Input: dimensioned drawing with shaded views. Units: mm. Origin: part minimum x, y, z. Round coordinates to 2 decimals unless told otherwise and drop trailing zeros. Loops run counter-clockwise (first coordinate to the right, second up) from the corner with the lowest first, then second, coordinate; pieces in that order, holes last. Notation, with made-up numbers: M 23,14 L 69,14 A15 cw 69,24 Z; hole C 62,-22 d4. An arc over 180 degrees is marked long. Use one line per item in the form item = value. Start each with the question number.
Q1. Section query A-A, the plane z = 16.51. Output: boundary loops of the cut face in (x, y), and give its area (3 significant figures).
Q2. Section query B-B, the plane x = 35.56. Output: boundary loops of the cut face in (y, z), and give its area (3 significant figures).
Q3. Ray query, line 1 along X through (y, z) = (0.95, 16.51); line 2 along Z through (x, y) = (22, 1.8); line 3 along X through (y, z) = (0.55, 18.5). Return the intervals inside material, ascending.
Q4. Section query C-C, the plane y = 0.5. Output: boundary loops of the cut face in (x, z).
Q5. First-contact query: P1, Ø24.5, axis at x = 35.56, z = 16.51, coming from the +Y side. Flat tip, straight axial feed; report the tip coordinate or a pass-through.
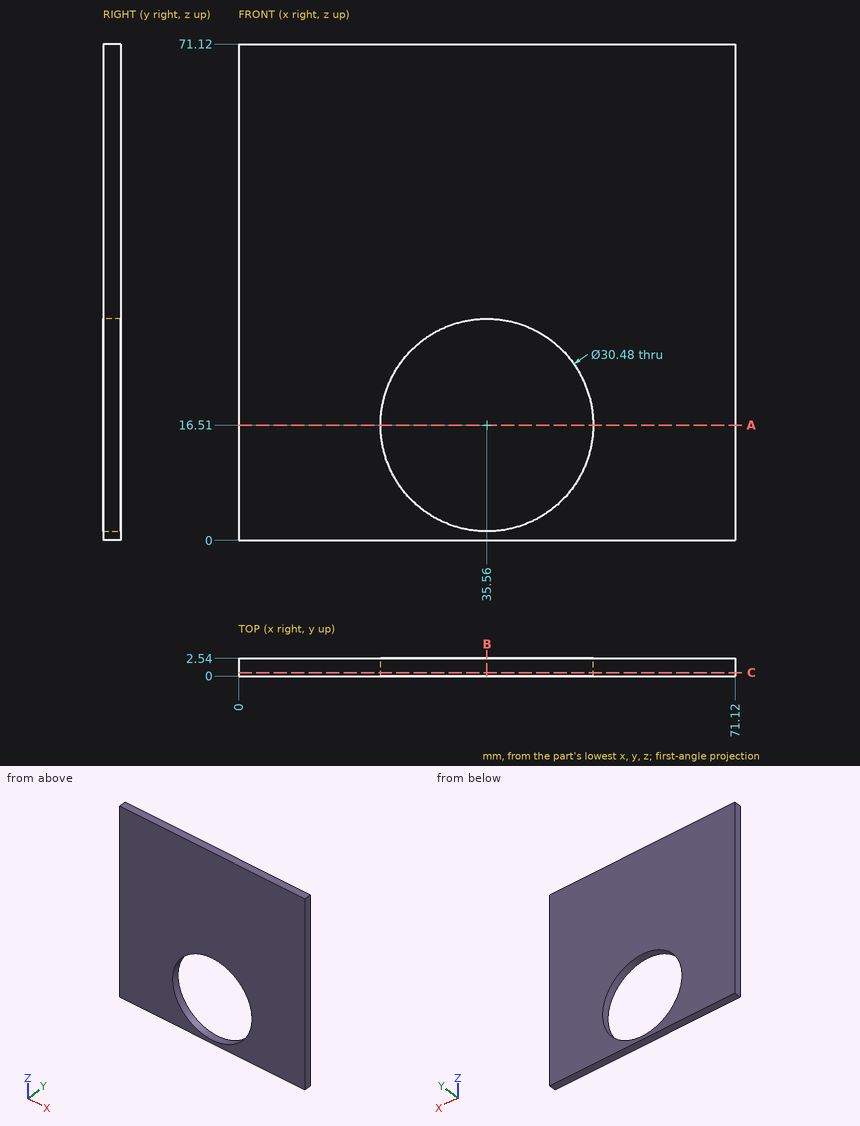
Results found:
q1.outline = M 0,0 L 20.32,0 L 20.32,2.54 L 0,2.54 Z; M 50.8,0 L 71.12,0 L 71.12,2.54 L 50.8,2.54 Z
q1.area = 103 mm²
q2.outline = M 0,0 L 2.54,0 L 2.54,1.27 L 0,1.27 Z; M 0,31.75 L 2.54,31.75 L 2.54,71.12 L 0,71.12 Z
q2.area = 103 mm²
q3.line_1 = 0 to 20.32, 50.8 to 71.12
q3.line_2 = 0 to 9.55, 23.47 to 71.12
q3.line_3 = 0 to 20.45, 50.67 to 71.12
q4.outline = M 0,0 L 71.12,0 L 71.12,71.12 L 0,71.12 Z; hole C 35.56,16.51 d30.48
q5.P1 = through
